Job drawing, mm, ordinate dimensions from the low corner. One solid piece. Give positions to 0.01 mm unless a question says otherwise; leave off trailing zeros. Loops run counter-clockwise (first coordinate to the right, second up) from the corner with the lowest first, then second, coordinate; pieces in that order, holes last. Notation, with made-up numbers: M 42.5,53 L 90.5,53 A23 ccw 90.5,69 Z; hole C 33.25,-33.75 d1. An arc over 180 degrees is marked long. Answer in a Markdown table with one row per item.
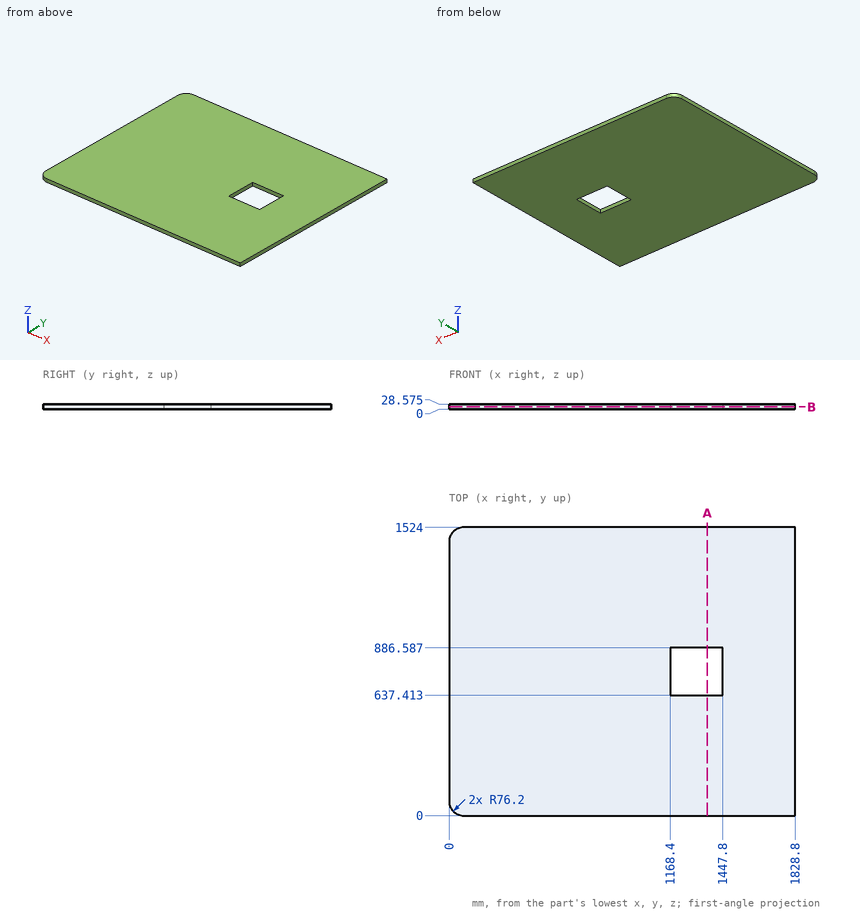
(1) Drill centre lines: line 1 along X through (y, z) = (682.5, 16); line 2 along Y through (x, z) = (1306, 25.25). Where is each one in solid material? Low to high.
Recorded:
| item | result |
|---|---|
| line 1 | x = 0 to 1168.4, 1447.8 to 1828.8 |
| line 2 | y = 0 to 637.41, 886.59 to 1524 |
(2) Saw through at A-A (x = 1365.5). Write the cut outline in (y, z) (3 decimals).
Recorded:
| item | result |
|---|---|
| outline | M 0,0 L 637.413,0 L 637.413,28.575 L 0,28.575 Z; M 886.587,0 L 1524,0 L 1524,28.575 L 886.587,28.575 Z |
(3) Pin check, flat tip, straight feed: pin 1 Ø2 at (y, z) = (160.5, 23.5) entering from -X. Stop position of the tip, or through.
Recorded:
| item | result |
|---|---|
| pin 1 | stops at x = 0 |
(4) Saw through at B-B (z = 13.25). Write the cut outline in (x, y), plus the area to 3 significant figures.
Recorded:
| item | result |
|---|---|
| outline | M 0,76.2 A76.2 ccw 76.2,0 L 1828.8,0 L 1828.8,1524 L 76.2,1524 A76.2 ccw 0,1447.8 Z; hole M 1168.4,637.41 L 1447.8,637.41 L 1447.8,886.59 L 1168.4,886.59 Z |
| area | 2,710,000 mm^2 |
